```python
from build123d import *

# Parameters (mm, degrees)
F0_R     = 34.162118
F0_R_2   = 26.03014
F1_DEPTH = 25.4
F2_W     = 82.366947
F2_H     = 88.6334
F3_DEPTH = 11.938
F5_DEPTH = 11.684


with BuildPart() as f1:
    # F0 (on Front) → F1 (new body)
    with BuildSketch(Plane.XZ):
        Circle(F0_R)
        Circle(F0_R_2, mode=Mode.SUBTRACT)
    extrude(amount=F1_DEPTH)

    # F2 (on Front) → F3 (join)
    with BuildSketch(Plane.XZ):
        with Locations((-67.186301, 6.906649)):
            Rectangle(F2_W, F2_H)
    extrude(amount=F3_DEPTH)

    # F4 (on Top) → F5 (join)
    with BuildSketch(Plane.XY):
        Polygon((-56.507535, -12.315094), (-33.903457, -25.42158), (-33.660881, -12.315094), align=None)
    extrude(amount=F5_DEPTH)


solid = f1.part
```
Verification items for the finished model (mm, model axes). A direction names the side the tool comes from. Round coordinates to 2 decimals unless told otherwise and drop trailing zeros. Write each loop counter-clockwise with the first axis right and the second up, starting at its lowest first coordinate (ties: lowest second). Pieces come first, ordered by that corner, then holes. Notation, with made-up numbers: (76, 75.25) - (106, 75.25) arc R6 ccw to (106, 82.25) - close; hole circle Ø4 at (15, 58). An arc over 180 degrees is marked (long way). Answer as a JSON object with one key per item and string values. Group by question number.
Q1. Section check C-C, the plane z = 16.5. Enter the section's corners in (x, y).
Q2. Tool access check on faces 1 (the flat face through (-43, -17, 11.684)), 2 (the flat face through (-41, -16, 0)). Record the directions out of +Z, -Z, +X, -X, +Y, -Y that give a thin tool (end or side, any length) a straight path to the whole face; none if there is none.
Q3. Section check D-D, the plane z = 36. Enter the section's corners in (x, y).
Q4. Go/stop test with flat-tipped pins: pin 1 Ø1.5 at (x, y) = (10, -10.5) entering from -Z; pin 2 Ø1 at (x, z) = (-62, 32) entering from +Y; pin 3 Ø4 at (x, y) = (-46.5, -21) entering from -Z; pin 4 Ø3 at (x, z) = (-52.5, 13) entering from -Y. Record where each tip stops, or that it passes through.
Q5. Mould release check, pull along Z, two halves, no side actions. Record for faces 3 (the flat face through (-68, -6, 51.223)), 4 (the flat face through (-26.003, -6, -30)), 5 (the flat face through (-68, -6, -37.41)), 6 (the cylindrical face through (24.045, -12.522, -9.97)): released by +Z, released by -Z, zero draft, split by the parting line, or undercut.
Q6. Thickness scan on line 1 (Z direction, x = 0, y = -8); line 2 (X direction, y = -9.75, z = 0). Record the ranges inside material, lowest first.
Q7. Section check A-A, the plane y = -3.25. Enter the section's corners in (x, z).
Q8. Section check B-B, the plane x = 0. Enter the section's corners in (y, z), plus the area to 3 significant figures.
Found:
{
 "1": {"outline": "(-108.37, -11.94) - (-29.91, -11.94) - (-29.91, -25.4) - (-20.13, -25.4) - (-20.13, 0) - (-108.37, 0) - close; (20.13, -25.4) - (29.91, -25.4) - (29.91, 0) - (20.13, 0) - close"},
 "2": {"face 1": "+Z, -X, -Y", "face 2": "-Z, -X, -Y"},
 "3": {"outline": "(-108.37, -11.94) - (-26, -11.94) - (-26, 0) - (-108.37, 0) - close"},
 "4": {"pin 1": "stops at z = -32.89", "pin 2": "stops at y = 0", "pin 3": "passes through", "pin 4": "stops at y = -15.06"},
 "5": {"face 3": "released by +Z", "face 4": "zero draft", "face 5": "released by -Z", "face 6": "undercut"},
 "6": {"line 1": "z = -34.16 to -26.03, 26.03 to 34.16", "line 2": "x = -108.37 to -26, 26.03 to 34.16"},
 "7": {"outline": "(-108.37, -37.41) - (-26, -37.41) - (-26, -22.16) arc R34.16 ccw (long way) to (-26, 22.16) - (-26, 51.22) - (-108.37, 51.22) - close; hole (-26, -1.19) arc R26.03 ccw (long way) to (-26, 1.19) - close"},
 "8": {"outline": "(-25.4, -34.16) - (0, -34.16) - (0, -26.03) - (-25.4, -26.03) - close; (-25.4, 26.03) - (0, 26.03) - (0, 34.16) - (-25.4, 34.16) - close", "area": "413 mm^2"}
}
